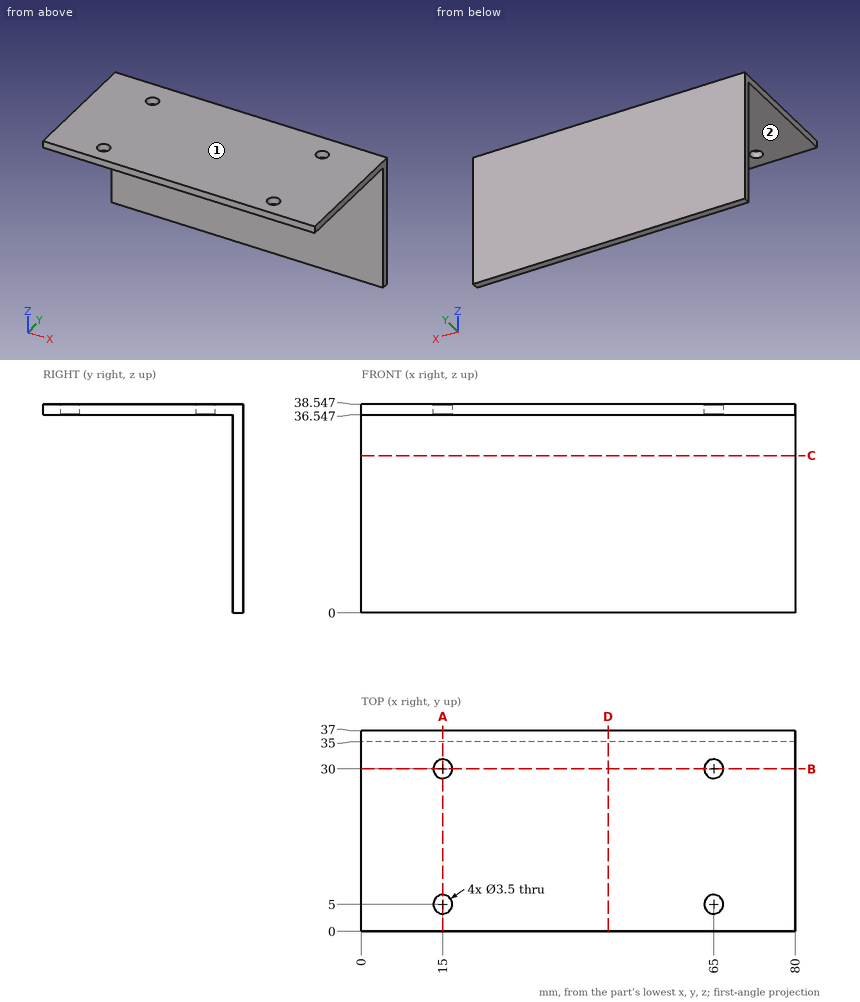
The figure shows three views and two pictorial views of one solid part (mm, origin at its lowest corner). Answer the questions. A direction names the side the tool comes from. Coordinates: 2 decimals unless noted, no trailing zeros. Write each loop counter-clockwise with the first axis right and the second up, starting at its lowest first coordinate (ties: lowest second). Pieces come first, ordered by that corner, then holes. Notation, with made-up numbers: M 50,18 L 57,18 A22 ccw 57,39 Z; hole C 74.25,5 d3. An arc over 180 degrees is marked long. Answer as CSV lines item,"result". Start each with the question number.
Item 1: Section C-C on z = 29 is taken. Write down the section's boundary in (x, y), and give its area (3 significant figures).
Item 2: Section B-B on y = 30 is taken. Write down the section's boundary in (x, z).
Item 3: Flat-ended cylindrical pins translate along their axes: P1, Ø3, axis at x = 69.5, y = 21, coming from the -Z side; P2, Ø5.5, axis at x = 15, y = 30, coming from the +Z side. Find the tip coordinate at first contact, or state that the pin passes through.
Item 4: A tool of negligible diameter and unlimited length cuts with its end or side. For the marked faces 1 and 2, from which of +Z, -Z, +X, -X, +Y, -Y can it reach the whole face along a straight path? Write none if from no direction.
Item 5: Consider L1, parallel to Y at x = 65, z = 37; L2, parallel to Y at x = 76, z = 35; L3, parallel to Z at x = 10.5, y = 20.5. Determine where each line is inside the solid, lowest interval first.
Item 6: Section A-A on x = 15 is taken. Write down the section's boundary in (y, z).
Item 7: Section D-D on x = 45.5 is taken. Write down the section's boundary in (y, z).
Checks:
1,outline,"M 0,35 L 80,35 L 80,37 L 0,37 Z"
1,area,"160 mm²"
2,outline,"M 0,36.55 L 13.25,36.55 L 13.25,38.55 L 0,38.55 Z; M 16.75,36.55 L 63.25,36.55 L 63.25,38.55 L 16.75,38.55 Z; M 66.75,36.55 L 80,36.55 L 80,38.55 L 66.75,38.55 Z"
3,P1,"stops at z = 36.55"
3,P2,"stops at z = 38.55"
4,face 1,"+Z, +X, -X, +Y, -Y"
4,face 2,"-Z, +X, -X, -Y"
5,L1,"y = 0 to 3.25, 6.75 to 28.25, 31.75 to 37"
5,L2,"y = 35 to 37"
5,L3,"z = 36.55 to 38.55"
6,outline,"M 0,36.55 L 3.25,36.55 L 3.25,38.55 L 0,38.55 Z; M 6.75,36.55 L 28.25,36.55 L 28.25,38.55 L 6.75,38.55 Z; M 31.75,36.55 L 35,36.55 L 35,0 L 37,0 L 37,38.55 L 31.75,38.55 Z"
7,outline,"M 0,36.55 L 35,36.55 L 35,0 L 37,0 L 37,38.55 L 0,38.55 Z"
